Autodesk Inventor part; units mm, degrees
ref_plane "YZ Plane" through (0, 0, 0) normal (1, 0, 0) x (0, 1, 0)
ref_plane "XZ Plane" through (0, 0, 0) normal (0, 1, 0) x (-1, 0, 0)
ref_plane "XY Plane" through (0, 0, 0) normal (0, 0, 1) x (1, 0, 0)
sketch "Sketch1" plane through (0, 0, 0) normal (0, 1, 0) x (-1, 0, 0)
  line L0 (0, 0) -> (50, 0)
  line L1 (0, 0) -> (0, -7)
  line L2 (0, -7) -> (6, -7)
  line L3 (6, -7) -> (6, -5)
  line L4 (6, -5) -> (8, -5)
  line L5 (8, -5) -> (8, -9)
  line L6 (8, -9) -> (32, -9)
  line L7 (32, -9) -> (32, -11.5)
  line L8 (32, -11.5) -> (35, -11.5)
  line L9 (35, -11.5) -> (35, -14.3615)
  line L10 (35, -14.3615) -> (38, -14.3615)
  line L11 (38, -14.3615) -> (38, -11.5)
  line L12 (38, -11.5) -> (45.2698, -11.5)
  line L13 (45.2698, -11.5) -> (45.2698, -7)
  line L14 (45.2698, -7) -> (50, -7)
  line L15 (50, -7) -> (50, 0)
  line L16 (0, 0) -> (27.4762, 0)
  line L17 (27.4762, 0) -> (27.4762, -2)
  line L18 (27.4762, -2) -> (0, -2)
  line L19 (0, -2) -> (0, 0)
  point P0 (7, -5)
  point P1 (32, -10.25)
  dimension "d0" = 50
  dimension "d1" = 7
  dimension "d2" = 6
  dimension "d3" = 2
  dimension "d4" = 5
  dimension "d6" = 24
  dimension "d7" = 3
  dimension "d8" = 3
  dimension "d9" = 11.5
  dimension "d10" = 9
  dimension "d12" = 2
revolve "Revolution1" add sketch "Sketch1" angle 360 about axis through (0, 0, 0) along (-1, 0, 0) contours L0 L15 L14 L13 L12 L11 L10 L9 L8 L7 L6 L5 L4 L3 L2 L1 L18 L17
sketch "Sketch2" plane through (0, 0, 0) normal (0, 1, 0) x (-1, 0, 0)
  line L0 (50, -7) -> (50, 7)
  line L1 (45.2698, -7) -> (45.2698, 7)
  circle A0 centre (54.2556, 0) radius 3.25
  arc A1 (54.2556, -4.7218) -> (54.2556, 4.7218) centre (54.2556, 0) ccw
  line L2 (54.2556, 4.7218) -> (50, 4.7218)
  line L3 (54.2556, -4.7218) -> (50, -4.7218)
  point P0 (0, 0)
  dimension "d13" = 6.5
extrude "Extrusion1" add sketch "Sketch2" along normal mid plane 4
fillet "Fillet1" radius 2 1 edges at (-50, 0, 7)
sketch "Sketch3" plane through (-45.2698, 0, 0) normal (-1, 0, 0) x (0, 0, 1)
  circle A0 centre (0, 0) radius 11.5
  circle A1 centre (0, 0) radius 2
  line L0 (11.5, 0) -> (5.75, -9.9593)
  line L1 (5.75, -9.9593) -> (-5.75, -9.9593)
  line L2 (-5.75, -9.9593) -> (-11.5, 0)
  line L3 (-11.5, 0) -> (-5.75, 9.9593)
  line L4 (-5.75, 9.9593) -> (5.75, 9.9593)
  line L5 (5.75, 9.9593) -> (11.5, 0)
  point P0 (-11.5, 0)
  point P1 (-11.5, 0)
  point P2 (-5.75, -9.9593)
  point P3 (-5.75, -9.9593)
extrude "Extrusion2" cut sketch "Sketch3" against normal up to surface (7.2698 mm away) contours L5 A0 | A0 L0 | L4 A0 | A0 L1 | L3 A0 | A0 L2
thread "Thread1"
properties part number "100MMshockUpper"
Build history of the part. All positions in model axes, mm. A direction names the side the tool comes from. Give positions to 0.01 mm unless a question says otherwise; leave off trailing zeros. Order: outer loops, then holes, each group sorted by start corner. A loop starts at its lowest first (then second) coordinate and runs counter-clockwise, first axis right, second up. Notation, with made-up numbers: M -3.5,53 L 17.5,53 A14 ccw 17.5,75 Z; hole C -33.5,-37 d2. An arc over 180 degrees is marked long. Put each result on its own line as item: value.
Item 1: Cut at C-C on x = -28.5. Write the cut outline in (y, z).
Results are:
outline: C 0,0 d18
Item 2: Cut at D-D on x = -12.5. Write the cut outline in (y, z).
Results are:
outline: C 0,0 d18; hole C 0,0 d4
Item 3: Wall check: probe 1 along Y at (x, z) = (-17, 0); probe 2 along X at (y, z) = (5, 9). Give the ranges that are in metal, low to high.
Results are:
probe 1: -9 to -2, 2 to 9
probe 2: -38 to -32
Item 4: Pull direction Z, two halves, no side cores. Call faces 5 (the face through (-14, -2, 0)), 6 (the face through (-51, -2, -2)), 7 (the face through (-20.168, -8.923, 1.172)), 8 (the face through (-27.476, 0, 0)): +Z half, -Z half, draft (parallel to the pull), parting line (faces both ways), or undercut.
Results are:
face 5: undercut
face 6: draft
face 7: parting line
face 8: undercut
Item 5: Cut at B-B on z = -8.25. Write the cut outline in (x, y), then the cut area to 3 significant figures.
Results are:
outline: M -45.27,-5.63 L -38,-5.63 L -38,-11.76 L -35,-11.76 L -35,-8.01 L -32,-8.01 L -32,-3.6 L -8,-3.6 L -8,3.6 L -32,3.6 L -32,8.01 L -35,8.01 L -35,11.76 L -38,11.76 L -38,5.63 L -45.27,5.63 Z
area: 373 mm2
Item 6: Cut at A-A on x = -55. Write the cut outline in (y, z), then the cut area to 3 significant figures.
Results are:
outline: M -2,-4.66 L 2,-4.66 L 2,-3.16 L -2,-3.16 Z; M -2,3.16 L 2,3.16 L 2,4.66 L -2,4.66 Z
area: 12.0 mm2
Item 7: Drop flat-ended pins along their axis: pin 1 Ø4.5 at (x, z) = (-53, -0.5) entering from +Y; pin 2 Ø1.2 at (x, y) = (-52, -0.5) entering from +Z; pin 3 Ø7.5 at (x, z) = (-54.26, 0) entering from -Y. Give the stop position or say it passes through.
Results are:
pin 1: y = 2
pin 2: z = 4.72
pin 3: y = -2
Item 8: Which spindle directions (+Z, -Z, +X, -X, +Y, -Y) get a long thin tool onto all of the face, cutting with end or side? Do faces 1 (the face through (-41.686, -5.049, -8.585)), 2 (the face through (-3.042, 2.681, -6.466)), 3 (the face through (-42, -9.959, 0)), 4 (the face through (-7.01, 4.88, 1.08)). Say none if no direction does.
Results are:
face 1: -Z, -X, -Y
face 2: +X
face 3: +Z, -Z, -X, -Y
face 4: none
